Build history of the part. All positions in model axes, mm. Give positions to 0.01 mm unless a question says otherwise; leave off trailing zeros. Order: outer loops, then holes, each group sorted by start corner. A loop starts at its lowest first (then second) coordinate and runs counter-clockwise, first axis right, second up. Notation, with made-up numbers: M 87.5,-22.75 L 109.5,-22.75 A23 cw 109.5,-7.75 Z; hole C 72,-14 d8. An arc over 180 degrees is marked long. Answer as CSV lines item,"result".
from build123d import *
from build123d.topology import SkipClean

# Parameters (mm, degrees)
SKETCH1_R                = 100
BOSS_EXTRUDE1_DEPTH      = 6.35
BOSS_EXTRUDE2_DEPTH      = 14.986
BOSS_EXTRUDE2_DEPTH_BACK = 76.128786138
SKETCH3_R                = 100
SKETCH3_R_2              = 94.92
BOSS_EXTRUDE3_DEPTH      = 5.842
CIRPATTERN1_COUNT        = 4
SKETCH29_W               = 5.08
SKETCH29_H               = 12.7
BOSS_EXTRUDE4_DEPTH      = 6.35
CIRPATTERN2_COUNT        = 4
CUT_EXTRUDE3_DEPTH       = 6.35
CUT_EXTRUDE4_START       = -9.144
CUT_EXTRUDE4_DEPTH       = 9.144
CIRPATTERN3_COUNT        = 4
BOSS_EXTRUDE6_DEPTH      = 12.7
CIRPATTERN4_COUNT        = 4
SKETCH34_W               = 25.4
SKETCH34_H               = 132.842
CUT_EXTRUDE5_DEPTH       = 7.62
CIRPATTERN5_COUNT        = 4
CUT_EXTRUDE6_START       = -88.9
CUT_EXTRUDE6_DEPTH       = 88.9


with BuildPart() as part:
    # Sketch1 → Boss-Extrude1 (new body)
    with BuildSketch(Plane(origin=(0, 0, 0), x_dir=(1, 0, 0), z_dir=(0, 1, 0))):
        with Locations(Location((0, 0, 0), (0, 0, 270))):
            Circle(SKETCH1_R)
    extrude(amount=BOSS_EXTRUDE1_DEPTH)

    # Sketch2 → Boss-Extrude2 (add, two sides: drawn at the far end of the back side and taken through both)
    with BuildSketch(Plane(origin=(0, 6.35, 0), x_dir=(1, 0, 0), z_dir=(0, 1, 0)).offset(-BOSS_EXTRUDE2_DEPTH_BACK)):
        with BuildLine():
            Line((70.138113747, -88.098625989), (79.118369868, -79.118369868))
            Line((79.118369868, -79.118369868), (88.098625989, -70.138113747))
            Line((88.098625989, -70.138113747), (79.118369868, -61.157857626))
            ThreePointArc((79.118369868, -61.157857626), (70.710678119, -70.710678119), (61.157857626, -79.118369868))
            Line((61.157857626, -79.118369868), (70.138113747, -88.098625989))
        make_face()
        with BuildLine():
            ThreePointArc((61.157857626, 79.118369868), (70.710678119, 70.710678119), (79.118369868, 61.157857626))
            Line((79.118369868, 61.157857626), (88.098625989, 70.138113747))
            Line((88.098625989, 70.138113747), (79.118369868, 79.118369868))
            Line((79.118369868, 79.118369868), (70.138113747, 88.098625989))
            Line((70.138113747, 88.098625989), (61.157857626, 79.118369868))
        make_face()
        with BuildLine():
            Line((-88.098625989, 70.138113747), (-79.118369868, 61.157857626))
            ThreePointArc((-79.118369868, 61.157857626), (-70.710678119, 70.710678119), (-61.157857626, 79.118369868))
            Line((-61.157857626, 79.118369868), (-70.138113747, 88.098625989))
            Line((-70.138113747, 88.098625989), (-79.118369868, 79.118369868))
            Line((-79.118369868, 79.118369868), (-88.098625989, 70.138113747))
        make_face()
        with BuildLine():
            Line((-79.118369868, -61.157857626), (-88.098625989, -70.138113747))
            Line((-88.098625989, -70.138113747), (-79.118369868, -79.118369868))
            Line((-79.118369868, -79.118369868), (-70.138113747, -88.098625989))
            Line((-70.138113747, -88.098625989), (-61.157857626, -79.118369868))
            ThreePointArc((-61.157857626, -79.118369868), (-70.710678119, -70.710678119), (-79.118369868, -61.157857626))
        make_face()
    extrude(amount=BOSS_EXTRUDE2_DEPTH + BOSS_EXTRUDE2_DEPTH_BACK)

    # Sketch3 → Boss-Extrude3 (add)
    with BuildSketch(Plane(origin=(0, 6.35, 0), x_dir=(1, 0, 0), z_dir=(0, 1, 0))):
        Circle(SKETCH3_R)
        with Locations(Location((0, 0, 0), (0, 0, 270))):
            Circle(SKETCH3_R_2, mode=Mode.SUBTRACT)
    extrude(amount=BOSS_EXTRUDE3_DEPTH)

    # Sweep1: sweep along a curve in space
    with BuildLine() as sweep1_path:
        Line((0, 0, 0), (-70.138113747, -53.268786138, -70.138113747))
    # 3DSketch4 → Sweep1 (sweep)
    with BuildSketch(Plane(origin=(-68.342062523, -59.618786138, -71.934164971), x_dir=(-0.262612865719444, 0.9284766908852601, 0.262612865719444), z_dir=(0.7071067811865448, -1.540105097113694e-15, 0.7071067811865502))):
        Polygon((0, 0), (1.886664636, 4.71666159), (13.67831861, 0), (11.791653974, -4.71666159), align=None)
    sweep1 = sweep(path=sweep1_path.line)

    # CirPattern1: Sweep1 ×4 about axis
    cirpattern1_axis = Axis((0, 0, 0), (0, 1, 0))
    for i in range(1, CIRPATTERN1_COUNT):
        add(sweep1.rotate(cirpattern1_axis, i * 360 / CIRPATTERN1_COUNT))

    # Sketch29 → Boss-Extrude4 (add)
    with BuildSketch(Plane(origin=(70.138113747, 0, 70.138113747), x_dir=(0.7071067811865501, 0, -0.7071067811865449), z_dir=(0.7071067811865449, 0, 0.7071067811865501))):
        with Locations((0, -53.268786138)):
            Rectangle(SKETCH29_W, SKETCH29_H)
    boss_extrude4 = extrude(amount=BOSS_EXTRUDE4_DEPTH)

    # CirPattern2: Boss-Extrude4 ×4 about axis
    cirpattern2_axis = Axis((0, 0, 0), (0, 1, 0))
    for i in range(1, CIRPATTERN2_COUNT):
        add(boss_extrude4.rotate(cirpattern2_axis, i * 360 / CIRPATTERN2_COUNT))

    # Sketch30 → Cut-Extrude3 (cut)
    with BuildSketch(Plane(origin=(0, 6.35, 0), x_dir=(1, 0, 0), z_dir=(0, 1, 0))):
        with BuildLine():
            Line((-10.1569893, -6.564886852), (-68.764267193, -65.172164744))
            ThreePointArc((-68.764267193, -65.172164744), (-94.741413859, 0), (-68.764267193, 65.172164744))
            Line((-68.764267193, 65.172164744), (-10.1569893, 6.564886852))
            Line((-10.1569893, 6.564886852), (-3.592102448, 0))
            Line((-3.592102448, 0), (-10.1569893, -6.564886852))
        make_face()
        with BuildLine():
            Line((-6.564886852, -10.1569893), (-65.172164744, -68.764267193))
            ThreePointArc((-65.172164744, -68.764267193), (0, -94.741413859), (65.172164744, -68.764267193))
            Line((65.172164744, -68.764267193), (6.564886852, -10.1569893))
            Line((6.564886852, -10.1569893), (0, -3.592102448))
            Line((0, -3.592102448), (-6.564886852, -10.1569893))
        make_face()
        with BuildLine():
            Line((-6.564886852, 10.1569893), (-65.172164744, 68.764267193))
            ThreePointArc((-65.172164744, 68.764267193), (0, 94.741413859), (65.172164744, 68.764267193))
            Line((65.172164744, 68.764267193), (6.564886852, 10.1569893))
            Line((6.564886852, 10.1569893), (0, 3.592102448))
            Line((0, 3.592102448), (-6.564886852, 10.1569893))
        make_face()
        with BuildLine():
            Line((10.1569893, 6.564886852), (68.764267193, 65.172164744))
            ThreePointArc((68.764267193, 65.172164744), (94.741413859, 0), (68.764267193, -65.172164744))
            Line((68.764267193, -65.172164744), (10.1569893, -6.564886852))
            Line((10.1569893, -6.564886852), (3.592102448, 0))
            Line((3.592102448, 0), (10.1569893, 6.564886852))
        make_face()
    extrude(amount=-CUT_EXTRUDE3_DEPTH, mode=Mode.SUBTRACT)

    # Sketch32 → Cut-Extrude4 (cut)
    with BuildSketch(Plane(origin=(0, 21.336, 0), x_dir=(1, 0, 0), z_dir=(0, 1, 0)).offset(CUT_EXTRUDE4_START)):
        with BuildLine():
            Line((79.118369868, 61.157857626), (88.098625989, 70.138113747))
            Line((88.098625989, 70.138113747), (70.138113747, 88.098625989))
            Line((70.138113747, 88.098625989), (61.157857626, 79.118369868))
            ThreePointArc((61.157857626, 79.118369868), (70.710678119, 70.710678119), (79.118369868, 61.157857626))
        make_face()
    cut_extrude4 = extrude(amount=CUT_EXTRUDE4_DEPTH, mode=Mode.SUBTRACT)

    # CirPattern3: Cut-Extrude4 ×4 about axis
    cirpattern3_axis = Axis((0, 12.192, 0), (0, -1, 0))
    for i in range(1, CIRPATTERN3_COUNT):
        add(cut_extrude4.rotate(cirpattern3_axis, i * 360 / CIRPATTERN3_COUNT), mode=Mode.SUBTRACT)

    # Sketch33 → Boss-Extrude6 (add, symmetric)
    with BuildSketch(Plane(origin=(0, 0, 0), x_dir=(-0.7071067811865438, 0, -0.7071067811865513), z_dir=(0.7071067811865513, 0, -0.7071067811865438))):
        Polygon((-94.707359271, -49.941543909), (-94.707359271, 0), (-100, 0), (-100, -46.918786138), (-100, -69.778786138), (-99.1902717, -69.778786138), (-94.707359271, -69.778786138), (-94.707359271, -63.948606699), align=None)
    boss_extrude6 = extrude(amount=BOSS_EXTRUDE6_DEPTH, both=True)

    # CirPattern4: Boss-Extrude6 ×4 about axis
    cirpattern4_axis = Axis((0, 0, 0), (0, 1, 0))
    for i in range(1, CIRPATTERN4_COUNT):
        add(boss_extrude6.rotate(cirpattern4_axis, i * 360 / CIRPATTERN4_COUNT))

    # Sketch34 → Cut-Extrude5 (cut)
    with BuildSketch(Plane(origin=(79.118369868, 0, 79.118369868), x_dir=(0.7071067811865465, 0, -0.7071067811865486), z_dir=(0.7071067811865486, 0, 0.7071067811865465))):
        with Locations((0, -54.229)):
            Rectangle(SKETCH34_W, SKETCH34_H)
    cut_extrude5 = extrude(amount=-CUT_EXTRUDE5_DEPTH, mode=Mode.SUBTRACT)

    # CirPattern5: Cut-Extrude5 ×4 about axis
    cirpattern5_axis = Axis((0, 0, 0), (0, 1, 0))
    for i in range(1, CIRPATTERN5_COUNT):
        add(cut_extrude5.rotate(cirpattern5_axis, i * 360 / CIRPATTERN5_COUNT), mode=Mode.SUBTRACT)

    # Sketch35 → Cut-Extrude6 (cut)
    with SkipClean():  # the faces are left unmerged after this step: merging them gives an invalid solid
        with BuildSketch(Plane(origin=(0, 12.192, 0), x_dir=(1, 0, 0), z_dir=(0, 1, 0)).offset(CUT_EXTRUDE6_START)):
            with BuildLine():
                Line((-61.157857626, 79.118369868), (-64.749960074, 82.710472317))
                Line((-64.749960074, 82.710472317), (-82.710472317, 64.749960074))
                Line((-82.710472317, 64.749960074), (-79.118369868, 61.157857626))
                ThreePointArc((-79.118369868, 61.157857626), (-70.710678119, 70.710678119), (-61.157857626, 79.118369868))
            make_face()
            with BuildLine():
                Line((-64.749960074, -82.710472317), (-61.157857626, -79.118369868))
                ThreePointArc((-61.157857626, -79.118369868), (-70.710678119, -70.710678119), (-79.118369868, -61.157857626))
                Line((-79.118369868, -61.157857626), (-82.710472317, -64.749960074))
                Line((-82.710472317, -64.749960074), (-64.749960074, -82.710472317))
            make_face()
            with BuildLine():
                Line((61.157857626, -79.118369868), (64.749960074, -82.710472317))
                Line((64.749960074, -82.710472317), (82.710472317, -64.749960074))
                Line((82.710472317, -64.749960074), (79.118369868, -61.157857626))
                ThreePointArc((79.118369868, -61.157857626), (70.710678119, -70.710678119), (61.157857626, -79.118369868))
            make_face()
            with BuildLine():
                Line((79.118369868, 61.157857626), (82.710472317, 64.749960074))
                Line((82.710472317, 64.749960074), (64.749960074, 82.710472317))
                Line((64.749960074, 82.710472317), (61.157857626, 79.118369868))
                ThreePointArc((61.157857626, 79.118369868), (70.710678119, 70.710678119), (79.118369868, 61.157857626))
            make_face()
        extrude(amount=CUT_EXTRUDE6_DEPTH, mode=Mode.SUBTRACT)


solid = part.part
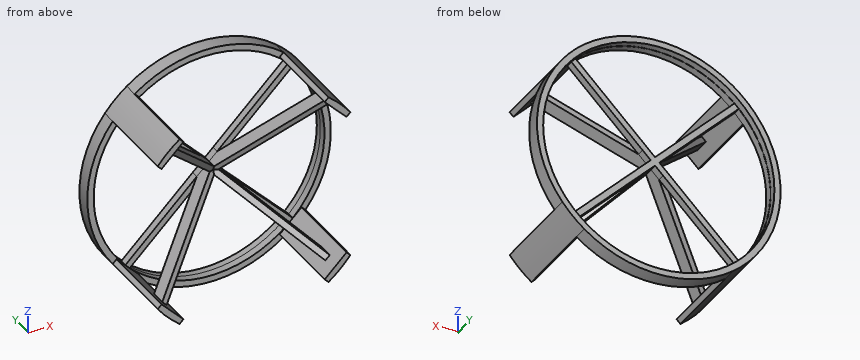
Item 1: Probe line 1 along X through (y, z) = (8.3, 0); line 2 along Z through (x, y) = (59.5, -35); line 3 along Z through (x, y) = (52, 4). List the from-to ranges inside material, lowest first. Write a range as from..to.
Geometry says:
line 1,"x = -100..-94.92, 94.92..100"
line 2,"z = -77.46..-74.44, 74.44..77.46"
line 3,"z = -85.42..-79.2, -55.59..-48.41, 48.41..55.59, 79.2..85.42"
Item 2: Band-saw the part on A-A (z = -55.5). Give the cut face in (x, y).
Geometry says:
outline,"M -83.19,0 L -76.78,0 L -76.78,6.35 L -77,6.35 L -77,12.19 L -83.19,12.19 Z; M -59.09,-49.87 L -51.91,-47.14 L -51.91,-34.44 L -59.09,-37.17 Z; M -59.09,0 L -51.91,0 L -51.91,6.35 L -59.09,6.35 Z; M 51.91,-47.14 L 59.09,-49.87 L 59.09,-37.17 L 51.91,-34.44 Z; M 51.91,0 L 59.09,0 L 59.09,6.35 L 51.91,6.35 Z; M 76.78,0 L 83.19,0 L 83.19,12.19 L 77,12.19 L 77,6.35 L 76.78,6.35 Z"
Item 3: Band-saw the part on B-B (x = 47). Give the cut face in (y, z).
Geometry says:
outline,"M -43.41,-50.59 L -30.71,-50.59 L -27.98,-43.41 L -40.68,-43.41 Z; M -43.41,50.59 L -40.68,43.41 L -27.98,43.41 L -30.71,50.59 Z; M 0,-88.27 L 12.19,-88.27 L 12.19,-82.47 L 6.35,-82.47 L 6.35,-82.26 L 0,-82.26 Z; M 0,-50.59 L 6.35,-50.59 L 6.35,-43.41 L 0,-43.41 Z; M 0,43.41 L 6.35,43.41 L 6.35,50.59 L 0,50.59 Z; M 0,82.26 L 6.35,82.26 L 6.35,82.47 L 12.19,82.47 L 12.19,88.27 L 0,88.27 Z"
Item 4: Band-saw the part on C-C (y = -47.5). State how many separate pieces and enclosed holes the cut face has, and give its area (3 significant figures).
Geometry says:
separate pieces,"4"
enclosed holes,"0"
area,"878 mm2"
Item 5: Drop flat-ended pins along their axis: pin 1 (4 mm diameter, centred on x = 66, y = 1.5, fed in from -Z); pin 2 (25 mm diameter, centred on x = 90, z = -21.5, fed in from -Y); pin 3 (8 mm diameter, centred on y = -20.5, z = -59, fed in from +X). Give the stop position or say it passes through.
Geometry says:
pin 1,"stops at z = -76.84"
pin 2,"stops at y = 0"
pin 3,"stops at x = 79.12"
